Read the model definition and answer for the solid it produces. Units are mm, in the model's axes. A direction names the side the tool comes from. Give positions to 0.01 mm unless a question says otherwise; leave off trailing zeros. Loops run counter-clockwise (first coordinate to the right, second up) from the corner with the lowest first, then second, coordinate; pieces in that order, holes last.
(1) Find section C-C, the plane z = 9. Write down the section's boundary in (x, y).
(2) Find section B-B, the plane x = 8. Write down the section's boundary in (y, z).
(3) Find section D-D, the plane y = -15.5. Write down the section's boundary in (x, z), then the cut area to 3 significant figures.
(4) Find section A-A, the plane y = -10. Write down the section's boundary in (x, z).
(5) Which of the six approach directions +Z, -Z, +X, -X, +Y, -Y give full straight-line access (tool end or side, diameter ignored) to faces 1 (the face through (8, -10, -16)), 2 (the face through (8, -35, -23)), 3 (the face through (8, -38, 6)), 4 (the face through (8, -18, 4)), 5 (the face through (7.8, 0, -16.2))?
(6) Each of these flat-tipped pins is pushed along its axis until it touches: P1, Ø1.9, axis at x = 16, z = 9, coming from the -Y side; P2, Ø4, axis at x = 0, z = 9, coming from the +Y side; P3, Ø13, axis at x = 4.5, y = -6.5, coming from the +Z side; P4, Ø8, axis at x = 5.5, y = -6.5, coming from the -Z side. Where does it stop, or does it pass through?
(7) Straight lines are drawn through the part: probe 1 along X at (y, z) = (-36, -25); probe 2 along X at (y, z) = (-15.5, -5); probe 3 along Z at (x, y) = (14.75, -6). For each, find the intervals that lie inside material, in ascending order.
(8) Determine the mould class of faces 6 (the face through (0, -10, -8)), 7 (the face through (8, -17, -20)), 8 (the face through (-1.972, -8.145, -5.183)), 9 (the face through (-4, -19, -8)) for opening direction Z: pulls with the +Z half, pulls with the -Z half, needs draft (parallel to the pull), parting line crosses it, or undercut.
```python
from build123d import *

# Parameters (mm, degrees)
SKETCH_1_W          = 16
SKETCH_1_H          = 16
EXTRUDE_1_DEPTH     = 20
SKETCH_2_W          = 24
SKETCH_2_H          = 24
EXTRUDE_4_DEPTH     = 10
SKETCH_3_W          = 4
SKETCH_3_H          = 3
EXTRUDE_6_DEPTH     = 24
SKETCH_5_R          = 1.6
CUT_EXTRUDE_1_DEPTH = 24
SKETCH_6_R          = 2.2
CUT_EXTRUDE_2_DEPTH = 25


with BuildPart() as part:
    # 草图1 → 凸台-拉伸1 (new body)
    with BuildSketch(Plane(origin=(0, 0, 0), x_dir=(1, 0, 0), z_dir=(0, 1, 0))):
        Polygon((-4, 20), (-4, 16), (-4, -4), (16, -4), (20, -4), (20, 0), (20, 20), (0, 20), align=None)
        with Locations((8, 8)):
            Rectangle(SKETCH_1_W, SKETCH_1_H, mode=Mode.SUBTRACT)
    extrude(amount=-EXTRUDE_1_DEPTH)

    # 草图2 → 凸台-拉伸4 (add)
    with BuildSketch(Plane.XZ.offset(20)):
        with Locations((8, -8)):
            Rectangle(SKETCH_2_W, SKETCH_2_H)
    extrude(amount=EXTRUDE_4_DEPTH)

    # 草图3 → 凸台-拉伸6 (add)
    with BuildSketch(Plane.ZY.offset(4)):
        with Locations((10, -36.5)):
            Rectangle(SKETCH_3_W, SKETCH_3_H)
        with BuildLine():
            Line((4, -35), (4, -30))
            Line((4, -30), (-8.000000062, -30))
            ThreePointArc((-8.000000062, -30), (-2.343145773, -32.343145728), (0, -38))
            Line((0, -38), (8, -38))
            Line((8, -38), (8, -35))
            Line((8, -35), (4, -35))
        make_face()
        with BuildLine():
            ThreePointArc((-16, -38), (-13.656854272, -32.343145773), (-8.000000062, -30))
            Line((-8.000000062, -30), (-20, -30))
            Line((-20, -30), (-20, -35))
            Line((-20, -35), (-24, -35))
            Line((-24, -35), (-24, -38))
            Line((-24, -38), (-16, -38))
        make_face()
        with Locations((-26, -36.5)):
            Rectangle(SKETCH_3_W, SKETCH_3_H)
    extrude(amount=-EXTRUDE_6_DEPTH)

    # 草图5 → 切除-拉伸1 (cut)
    with BuildSketch(Plane.XZ.offset(38)):
        with Locations(Location((8, 9, 0), (0, 0, 270))):
            Circle(SKETCH_5_R)
        with Locations(Location((16, 9, 0), (0, 0, 270))):
            Circle(SKETCH_5_R)
        with Locations(Location((0, 9, 0), (0, 0, 90))):
            Circle(SKETCH_5_R)
        with Locations(Location((0, -25, 0), (0, 0, 270))):
            Circle(SKETCH_5_R)
        with Locations(Location((8, -25, 0), (0, 0, 270))):
            Circle(SKETCH_5_R)
        with Locations(Location((16, -25, 0), (0, 0, 270))):
            Circle(SKETCH_5_R)
    extrude(amount=-CUT_EXTRUDE_1_DEPTH, mode=Mode.SUBTRACT)

    # 草图6 → 切除-拉伸2 (cut, symmetric)
    with BuildSketch(Plane(origin=(0, 0, 0), x_dir=(0, 0, -1), z_dir=(1, 0, 0))):
        with Locations((12.280139498, -10)):
            Circle(SKETCH_6_R)
        with Locations((4, -10)):
            Circle(SKETCH_6_R)
    extrude(amount=CUT_EXTRUDE_2_DEPTH, both=True, mode=Mode.SUBTRACT)


solid = part.part
```
Entries:
1. outline: (-4, -38) - (-1.6, -38) - (-1.6, -35) - (-4, -35) - close; (1.6, -38) - (6.4, -38) - (6.4, -35) - (1.6, -35) - close; (9.6, -38) - (14.4, -38) - (14.4, -35) - (9.6, -35) - close; (17.6, -38) - (20, -38) - (20, -35) - (17.6, -35) - close
2. outline: (-38, -28) - (-35, -28) - (-35, -26.6) - (-38, -26.6) - close; (-38, -23.4) - (-35, -23.4) - (-35, -20) - (0, -20) - (0, -16) - (-20, -16) - (-20, 0) - (0, 0) - (0, 4) - (-35, 4) - (-35, 7.4) - (-38, 7.4) - (-38, 0) arc R8 cw to (-38, -16) - close; (-38, 10.6) - (-35, 10.6) - (-35, 12) - (-38, 12) - close
3. outline: (-4, -20) - (20, -20) - (20, 4) - (-4, 4) - close; hole (0, -16) - (16, -16) - (16, 0) - (0, 0) - close
3. area: 320 mm2
4. outline: (-4, -20) - (20, -20) - (20, -14.48) - (16, -14.48) - (16, -16) - (0, -16) - (0, -14.48) - (-4, -14.48) - close; (-4, -10.08) - (0, -10.08) - (0, -6.2) - (-4, -6.2) - close; (-4, -1.8) - (0, -1.8) - (0, 0) - (16, 0) - (16, -1.8) - (20, -1.8) - (20, 4) - (-4, 4) - close; (16, -10.08) - (20, -10.08) - (20, -6.2) - (16, -6.2) - close
5. face 1: +Y
5. face 2: -Z, +X, -X, +Y
5. face 3: +Z, -Z, +X, -X, -Y
5. face 4: +Z, +X, -X, +Y
5. face 5: +Z, -Z, +X, -X, +Y
6. P1: passes through
6. P2: stops at y = -35
6. P3: stops at z = 4
6. P4: stops at z = -20
7. probe 1: x = -4 to -1.6, 1.6 to 6.4, 9.6 to 14.4, 17.6 to 20
7. probe 2: x = -4 to 0, 16 to 20
7. probe 3: z = -20 to -16, 0 to 4
8. face 6: undercut
8. face 7: pulls with the -Z half
8. face 8: undercut
8. face 9: needs draft
